from build123d import *

# Parameters (mm, degrees)
F0_W      = 48
F0_H      = 25
F1_DEPTH  = 25
F3_DEPTH  = 25
F4_W      = 10
F4_H      = 33.5
F5_DEPTH  = 2.5
F6_W      = 10
F6_H      = 1.5
F6_H_2    = 2.5
F7_DEPTH  = 2
F8_W      = 10
F8_H      = 7.5
F8_H_2    = 2.5
F9_DEPTH  = 3
F10_W     = 8
F10_H     = 25
F11_DEPTH = 3
F12_R     = 1.6
F13_DEPTH = 3
F14_R     = 5
F15_R     = 2


with BuildPart() as f1:
    # F0 (on Front) → F1 (new body)
    with BuildSketch(Plane.XZ):
        Rectangle(F0_W, F0_H)
    extrude(amount=-F1_DEPTH)

    # F2 (on face) → F3 (cut, through all)
    with BuildSketch(Plane.XZ):
        with BuildLine():
            ThreePointArc((-22, -1.25), (-18.7049512883, -9.2049512883), (-10.75, -12.5))
            Line((-10.75, -12.5), (10.75, -12.5))
            ThreePointArc((10.75, -12.5), (18.7049512883, -9.2049512883), (22, -1.25))
            ThreePointArc((22, -1.25), (18.7049512883, 6.7049512883), (10.75, 10))
            Line((10.75, 10), (-10.75, 10))
            ThreePointArc((-10.75, 10), (-18.7049512883, 6.7049512883), (-22, -1.25))
        make_face()
        with BuildLine():
            Line((-22, -12.5), (-10.75, -12.5))
            ThreePointArc((-10.75, -12.5), (-18.7049512883, -9.2049512883), (-22, -1.25))
            Line((-22, -1.25), (-22, -12.5))
        make_face()
        with BuildLine():
            ThreePointArc((22, -1.25), (18.7049512883, -9.2049512883), (10.75, -12.5))
            Line((10.75, -12.5), (22, -12.5))
            Line((22, -12.5), (22, -1.25))
        make_face()
    extrude(amount=-F3_DEPTH, mode=Mode.SUBTRACT)

    # F4 (on face) → F5 (join, through all)
    with BuildSketch(Plane.XY.offset(12.5)):
        with Locations((0, 41.75)):
            Rectangle(F4_W, F4_H)
        with Locations((0, -16.75)):
            Rectangle(F4_W, F4_H)
    extrude(amount=-F5_DEPTH)

    # F6 (on face) → F7 (join)
    with BuildSketch(Plane.XZ.offset(33.5)):
        with Locations((0, 9.25)):
            Rectangle(F6_W, F6_H)
        with Locations((0, 11.25)):
            Rectangle(F6_W, F6_H_2)
    extrude(amount=F7_DEPTH)

    # F8 (on face) → F9 (join)
    with BuildSketch(Plane(origin=(0, 58.5, 0), x_dir=(-1, 0, 0), z_dir=(0, 1, 0))):
        with Locations((0, 6.25)):
            Rectangle(F8_W, F8_H)
        with Locations((0, 11.25)):
            Rectangle(F8_W, F8_H_2)
    extrude(amount=F9_DEPTH)

    # F10 (on face) → F11 (join)
    with BuildSketch(Plane(origin=(0, 0, -12.5), x_dir=(1, 0, 0), z_dir=(0, 0, -1))):
        with Locations((-28, -12.5)):
            Rectangle(F10_W, F10_H)
        with Locations((28, -12.5)):
            Rectangle(F10_W, F10_H)
    extrude(amount=-F11_DEPTH)

    # F12 (on face) → F13 (cut, through all)
    with BuildSketch(Plane(origin=(0, 0, -12.5), x_dir=(1, 0, 0), z_dir=(0, 0, -1))):
        with Locations((-27.5, -5)):
            Circle(F12_R)
        with Locations((-27.5, -20)):
            Circle(F12_R)
        with Locations((27.5, -20)):
            Circle(F12_R)
        with Locations((27.5, -5)):
            Circle(F12_R)
    extrude(amount=-F13_DEPTH, mode=Mode.SUBTRACT)

    # F14
    f14_edges = [f1.edges().sort_by_distance(p)[0] for p in [
        (-24, 12.5, 12.5),
        (24, 12.5, 12.5),
        (-5, 25, 11.25),
        (-5, 0, 11.25),
        (5, 0, 11.25),
        (5, 25, 11.25),
    ]]
    fillet(f14_edges, radius=F14_R)

    # F15
    f15_edges = [f1.edges().sort_by_distance(p)[0] for p in [
        (0, 61.5, 12.5),
        (0, -35.5, 12.5),
        (22, 12.5, -12.5),
        (-22, 12.5, -12.5),
        (-32, 12.5, -9.5),
        (32, 12.5, -9.5),
    ]]
    fillet(f15_edges, radius=F15_R)


solid = f1.part
Can you work these out from the model? Positions are in its coordinate system, mm. A direction names the side the tool comes from. Give positions to 0.01 mm unless a question says otherwise; leave off trailing zeros. Loops run counter-clockwise (first coordinate to the right, second up) from the corner with the lowest first, then second, coordinate; pieces in that order, holes last. Notation, with made-up numbers: M 51.5,74 L 102.5,74 A18 ccw 102.5,108 Z; hole C 73,-33.75 d7. An arc over 180 degrees is marked long. One line per item, written item: value. Start each with the question number.
1) If we section it at C-C, the plane x = -27.5: Write out the boundary of the cut face in (y, z).
2) If we section it at B-B, the plane y = 20: Write out the boundary of the cut face in (x, z), and give its area (3 significant figures).
3) If I drill on line 1 (Y direction, x = 27.5, z = -11.4); line 2 (X direction, y = 1.5, z = -6); line 3 (X direction, y = 5, z = -10.3), over which ranges is the centre line in solid material (lowest first)? Write a range as [from, to].
4) I'm going to push flat-ended pins straight in: pin 1 (2.5 mm diameter, centred on x = -0.5, y = 59.5, fed in from -Z); pin 2 (10 mm diameter, centred on y = 6.5, z = 3.5, fed in from -X); pin 3 (11 mm diameter, centred on x = -25, z = 1.5, fed in from -Y). Where does each tip first touch, or does it pass through?
5) On a 3-axis mill with a long thin cutter (end or side, diameter ignored), from which of +Z, -Z, +X, -X, +Y, -Y can I reach the whole of each face in a straight line? I mean faces 5 (the face through (27, 12, -9.5)), 6 (the face through (5, -20, 11)), 7 (the face through (-5, 49.2, 10.4)). Say none if no direction works.
6) If we section it at A-A, the plane z = -7.75: Write out the boundary of the cut face in (x, y), and give its area (3 significant figures).
7) If we section it at D-D, the plane x = -7: Write out the boundary of the cut face in (y, z).
8) Thinking about a two-plate mould opening in X: for faces 1 (the face through (0, 12, 10)), 2 (the face through (-28, 12, -12.5)), 3 (the face through (-22.57, 12.68, 11)), 4 (the face through (22.5, 12.68, 11.07)), which applies, +X half, -X half, draft (parallel to the pull), parting line (faces both ways), or undercut?
Completed:
1. outline: M 0,-12.5 L 3.4,-12.5 L 3.4,-9.5 L 0,-9.5 Z; M 6.6,-12.5 L 18.4,-12.5 L 18.4,-9.5 L 6.6,-9.5 Z; M 21.6,-12.5 L 25,-12.5 L 25,-9.5 L 21.6,-9.5 Z
2. outline: M -32,-12.5 L -29.1,-12.5 L -29.1,-9.5 L -30,-9.5 A2 ccw -32,-11.5 Z; M -25.9,-12.5 L -24,-12.5 A2 ccw -22,-10.5 L -22,-1.25 A11.25 cw -10.75,10 L 10.75,10 A11.25 cw 22,-1.25 L 22,-10.5 A2 ccw 24,-12.5 L 25.9,-12.5 L 25.9,-9.5 L 24,-9.5 L 24,7.5 A5 ccw 19,12.5 L -19,12.5 A5 ccw -24,7.5 L -24,-9.5 L -25.9,-9.5 Z; M 29.1,-12.5 L 32,-12.5 L 32,-11.5 A2 ccw 30,-9.5 L 29.1,-9.5 Z
2. area: 279 mm^2
3. line 1: y = [0, 3.4], [6.6, 18.4], [21.6, 25]
3. line 2: x = [-24, -22], [22, 24]
3. line 3: x = [-31.6, -29.1], [-25.9, -22], [22, 25.9], [29.1, 31.6]
4. pin 1: stops at z = 2.5
4. pin 2: stops at x = -24
4. pin 3: stops at y = 0
5. face 5: +Z, +X, +Y, -Y
5. face 6: +Z, -Z, +X, -Y
5. face 7: +Z, -Z, -X, +Y
6. outline: M -24,0 L -22,0 L -22,25 L -24,25 Z; M 22,0 L 24,0 L 24,25 L 22,25 Z
6. area: 100 mm^2
7. outline: M -1,10 L 26,10 L 26,12.5 L -1,12.5 Z
8. face 1: undercut
8. face 2: draft
8. face 3: -X half
8. face 4: +X half
